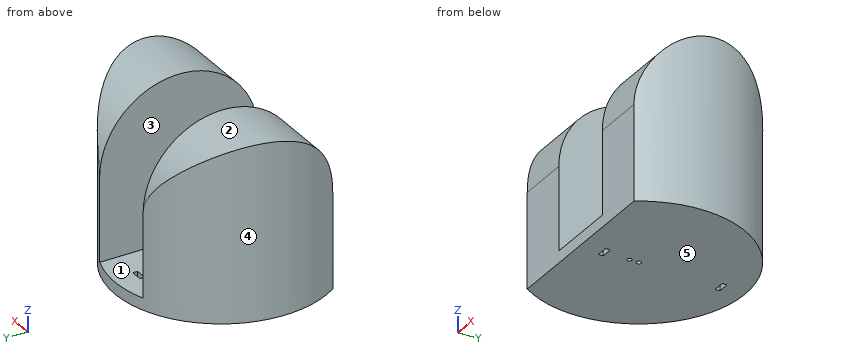
```python
from build123d import *

# Parameters (mm, degrees)
F1_DEPTH  = 5
F3_DEPTH  = 70
F5_DEPTH  = 29.352648758
F6_DEPTH  = 59.649351342
F7_W      = 5
F7_H      = 2
F8_DEPTH  = 5.0010001
F9_R      = 1
F10_DEPTH = 5.0010001


with BuildPart() as f1:
    # F0 (on Top) → F1 (new body)
    with BuildSketch(Plane.XY):
        with BuildLine():
            ThreePointArc((37.148351242, -24.5), (0, 44.5), (-37.148351242, -24.5))
            Line((-37.148351242, -24.5), (37.148351242, -24.5))
        make_face()
    extrude(amount=F1_DEPTH)

    # F2 (on face) → F3 (join)
    with BuildSketch(Plane.XY.offset(5)):
        with BuildLine():
            ThreePointArc((-15.148351242, 41.8422926553), (-42.2381488866, 14.0067404715), (-37.148351242, -24.5))
            Line((-37.148351242, -24.5), (-15.148351242, -24.5))
            Line((-15.148351242, -24.5), (-15.148351242, 41.8422926553))
        make_face()
        with BuildLine():
            Line((15.148351242, 41.8422926553), (15.148351242, -24.5))
            Line((15.148351242, -24.5), (37.148351242, -24.5))
            ThreePointArc((37.148351242, -24.5), (42.2381488866, 14.0067404715), (15.148351242, 41.8422926553))
        make_face()
    extrude(amount=F3_DEPTH)

    # F4 (on face) → F5 (cut, through all)
    with BuildSketch(Plane.YZ.offset(-15.148351242)):
        with BuildLine():
            ThreePointArc((-24.5, 40), (8.6711463276, 73.1711463276), (41.8422926553, 40))
            Line((41.8422926553, 40), (58.5, 40))
            Line((58.5, 40), (58.5, 90))
            Line((58.5, 90), (-45.5, 90))
            Line((-45.5, 90), (-45.5, 40))
            Line((-45.5, 40), (-24.5, 40))
        make_face()
    extrude(amount=-F5_DEPTH, mode=Mode.SUBTRACT)

    # F4 (on face) → F6 (cut, through all)
    with BuildSketch(Plane.YZ.offset(-15.148351242)):
        with BuildLine():
            ThreePointArc((-24.5, 40), (8.6711463276, 73.1711463276), (41.8422926553, 40))
            Line((41.8422926553, 40), (58.5, 40))
            Line((58.5, 40), (58.5, 90))
            Line((58.5, 90), (-45.5, 90))
            Line((-45.5, 90), (-45.5, 40))
            Line((-45.5, 40), (-24.5, 40))
        make_face()
    extrude(amount=F6_DEPTH, mode=Mode.SUBTRACT)

    # F7 (on face) → F8 (cut, through all)
    with BuildSketch(Plane.XY.offset(5)):
        Polygon((-2.5, 33.5), (0, 33.5), (2.5, 33.5), (2.5, 35.5), (-2.5, 35.5), align=None)
        with Locations((0, -14.5)):
            Rectangle(F7_W, F7_H)
    extrude(amount=-F8_DEPTH, mode=Mode.SUBTRACT)

    # F9 (on face) → F10 (cut, through all)
    with BuildSketch(Plane.XY.offset(5)):
        Circle(F9_R)
        with Locations((0, -4)):
            Circle(F9_R)
    extrude(amount=-F10_DEPTH, mode=Mode.SUBTRACT)


solid = f1.part
```
The listing builds one solid part. Answer for the finished solid, in the listing's coordinates (mm). Face numbers are marked on the shaded views. A direction names the side the tool comes from. Coordinates: 2 decimals unless noted, no trailing zeros. Loops run counter-clockwise (first coordinate to the right, second up) from the corner with the lowest first, then second, coordinate; pieces in that order, holes last. Notation, with made-up numbers: M 81,28.5 L 113,28.5 A9 ccw 113,45.5 Z; hole C 22,28 d3. An arc over 180 degrees is marked long. Answer as CSV lines item,"result". Start each with the question number.
(1) The part is cut by section D-D (x = 28). Give the vertices of the cut face in (y, z), and give its area (3 significant figures).
(2) For the marked faces 1 and 2, determine the directions among +Z, -Z, +X, -X, +Y, -Y from which every point of the face is accessible in a straight line to the end or side of a thin tool.
(3) The part is cut by section B-B (y = 19). Give the vertices of the cut face in (x, z).
(4) The part is cut by section A-A (z = 42). Give the vertices of the cut face in (x, y).
(5) Given pin 1 (1 mm diameter, centred on y = 13.5, z = 9.5, fed in from -X); pin 2 (10 mm diameter, centred on y = 21.5, z = 60, fed in from -X); pin 3 (5 mm diameter, centred on x = 13.5, z = 22.5, fed in from +Y); pin 4 (4 mm diameter, centred on x = -10, y = 27.5, fed in from -Z), each flat-ended and moving along its own axis, determine where each tip first touches the part or whether it passes through.
(6) The mould has two halves that part along X. Classify the marked faces 3, 4 and 5: pulls with the +X half, pulls with the -X half, needs draft (parallel to the pull), parting line crosses it, or undercut.
(7) The part is cut by section C-C (z = 7). Give the vertices of the cut face in (x, y), and give its area (3 significant figures).
(8) Find the intervals of material crossed by L1, parallel to Y at x = 0, z = 3.8; L2, parallel to Z at x = -6, y = 40.5; L3, parallel to X at y = 8, z = 43 (3 decimals), in increasing order. Write a range as [from, to].
Determined:
1,outline,"M -24.5,0 L 34.59,0 L 34.59,60.71 A33.17 ccw -24.5,40 Z"
1,area,"3,990 mm2"
2,face 1,"+Z, +Y, -Y"
2,face 2,"+Z, +X, -X"
3,outline,"M -40.24,0 L 40.24,0 L 40.24,71.52 L 15.15,71.52 L 15.15,5 L -15.15,5 L -15.15,71.52 L -40.24,71.52 Z"
4,outline,"M -37.19,-24.44 L -15.15,-24.44 L -15.15,41.78 L -15.31,41.78 A44.5 ccw Z; M 15.15,-24.44 L 37.19,-24.44 A44.5 ccw 15.31,41.78 L 15.15,41.78 Z"
5,pin 1,"x = -42.56"
5,pin 2,"x = -41.33"
5,pin 3,"y = 41.84"
5,pin 4,"z = 0"
6,face 3,"undercut"
6,face 4,"parting line crosses it"
6,face 5,"needs draft"
7,outline,"M -37.15,-24.5 L -15.15,-24.5 L -15.15,41.84 A44.5 ccw Z; M 15.15,-24.5 L 37.15,-24.5 A44.5 ccw 15.15,41.84 Z"
7,area,"3,110 mm2"
8,L1,"[-24.5, -15.5], [-13.5, -5], [-3, -1], [1, 33.5], [35.5, 44.5]"
8,L2,"[0, 5]"
8,L3,"[-43.775, -15.148], [15.148, 43.775]"
